from build123d import *

# Parameters (mm, degrees)
EXTRUDE_START            = -16
SKETCH_1_R               = 13
EXTRUDE_1_DEPTH          = 22
CUT_EXTRUDE_1_REACH      = 26.372
SKETCH_2_R               = 8
CUT_EXTRUDE_2_REACH      = 26.372
SKETCH_3_R               = 10
CUT_EXTRUDE_3_DEPTH      = 25.372115214
CUT_EXTRUDE_3_DEPTH_BACK = 25.372115214
SKETCH_4_R               = 3
SKETCH_4_R_2             = 2


with BuildPart() as part:
    # 草图1 → 凸台-拉伸1 (new body)
    with BuildSketch(Plane(origin=(0, 0, 0), x_dir=(1, 0, 0), z_dir=(0, 1, 0)).offset(EXTRUDE_START)):
        with Locations(Location((0, 0, 0), (0, 0, 270))):
            Circle(SKETCH_1_R)
    extrude(amount=EXTRUDE_1_DEPTH)

    # 草图2 → 切除-拉伸1 (cut, up to next)
    with BuildSketch(Plane(origin=(0, 0, 0), x_dir=(1, 0, 0), z_dir=(0, 1, 0)), mode=Mode.PRIVATE) as cut_extrude_1_sk1:
        with Locations(Location((0, 0, 0), (0, 0, 270))):
            Circle(SKETCH_2_R)
    cut_extrude_1_tool1 = extrude(cut_extrude_1_sk1.sketch, amount=CUT_EXTRUDE_1_REACH, mode=Mode.PRIVATE) & part.part
    add(cut_extrude_1_tool1.solids().sort_by_distance((0, 0, 0))[0], mode=Mode.SUBTRACT)

    # 草图3 → 切除-拉伸2 (cut, up to next)
    with BuildSketch(Plane(origin=(0, 0, 0), x_dir=(1, 0, 0), z_dir=(0, 1, 0)), mode=Mode.PRIVATE) as cut_extrude_2_sk1:
        with Locations(Location((0, 0, 0), (0, 0, 270))):
            Circle(SKETCH_3_R)
    cut_extrude_2_tool1 = extrude(cut_extrude_2_sk1.sketch, amount=-CUT_EXTRUDE_2_REACH, mode=Mode.PRIVATE) & part.part
    add(cut_extrude_2_tool1.solids().sort_by_distance((0, 0, 0))[0], mode=Mode.SUBTRACT)

    # 草图4 → 切除-拉伸3 (cut, two sides: drawn at the far end of the back side and taken through both)
    with BuildSketch(Plane.XY.offset(-CUT_EXTRUDE_3_DEPTH_BACK)):
        with Locations((0, -9)):
            Circle(SKETCH_4_R)
        with Locations((0, 3)):
            Circle(SKETCH_4_R_2)
    extrude(amount=CUT_EXTRUDE_3_DEPTH + CUT_EXTRUDE_3_DEPTH_BACK, mode=Mode.SUBTRACT)


solid = part.part
The listing builds one solid part. Answer for the finished solid, in the listing's coordinates (mm). A direction names the side the tool comes from. Round coordinates to 2 decimals unless told otherwise and drop trailing zeros. Order: outer loops, then holes, each group sorted by start corner. A loop starts at its lowest first (then second) coordinate and runs counter-clockwise, first axis right, second up. Notation, with made-up numbers: M 13,3.5 L 62,3.5 A16 cw 62,22.5 Z; hole C 1.25,76 d5. An arc over 180 degrees is marked long. Answer in a Markdown table with one row per item. Add a question column.
1) Determine the mould class of faces 3 (the face through (3, -7.89, 9.54)), 4 (the face through (-5, -5, 12)), 5 (the face through (0, 1, -10)) for opening direction Z: pulls with the +Z half, pulls with the -Z half, needs draft (parallel to the pull), parting line crosses it, or undercut.
2) Consider line 1 along Y through (x, z) = (0, 10.35); line 2 along X through (y, z) = (-9, -10.25); line 3 along X through (y, z) = (-4.25, 0). Determine where each line is inside the solid, lowest interval first. Write a range as from..to.
3) Flat-ended cylindrical pins translate along their axes: pin 1 Ø4 at (y, z) = (2.5, -10) entering from +X; pin 2 Ø4 at (x, y) = (5, -11.5) entering from +Z; pin 3 Ø1 at (x, y) = (8, -9) entering from -Z. Find the tip coordinate at first contact, or state that the pin passes through.
4) The part is cut by section B-B on y = -9. Determine the outline of the cut face in (x, z), plus the area to 3 significant figures.
5) Which of the six approach directions +Z, -Z, +X, -X, +Y, -Y give full straight-line access (tool end or side, diameter ignored) to faces 1 (the face through (8.2, 0, 0)), 2 (the face through (-3.06, 2.96, 7.39))?
6) The part is cut by section D-D on x = 4.75. Determine the outline of the cut face in (y, z).
7) The part is cut by section C-C on x = -1. Determine the outline of the cut face in (y, z).
8) The part is cut by section A-A on z = 0. Determine the outline of the cut face in (x, y), plus the area to 3 significant figures.
Findings below:
| question | item | result |
|---|---|---|
| 1 | face 3 | undercut |
| 1 | face 4 | parting line crosses it |
| 1 | face 5 | needs draft |
| 2 | line 1 | y = -16..-12, -6..1, 5..6 |
| 2 | line 2 | x = -8..-3, 3..8 |
| 2 | line 3 | x = -13..-10, 10..13 |
| 3 | pin 1 | stops at x = 10.25 |
| 3 | pin 2 | stops at z = 12.65 |
| 3 | pin 3 | stops at z = -10.62 |
| 4 | outline | M -3,-12.65 L -3,-9.54 A10 cw -3,9.54 L -3,12.65 A13 ccw Z; M 3,-12.65 A13 ccw 3,12.65 L 3,9.54 A10 cw 3,-9.54 Z |
| 4 | area | 180 mm² |
| 5 | face 1 | -Y |
| 5 | face 2 | +Y, -Y |
| 6 | outline | M -16,-12.1 L 6,-12.1 L 6,-6.44 L 0,-6.44 L 0,-8.8 L -16,-8.8 Z; M -16,8.8 L 0,8.8 L 0,6.44 L 6,6.44 L 6,12.1 L -16,12.1 Z |
| 7 | outline | M -16,-12.96 L -11.83,-12.96 L -11.83,-9.95 L -16,-9.95 Z; M -16,9.95 L -11.83,9.95 L -11.83,12.96 L -16,12.96 Z; M -6.17,-12.96 L 1.27,-12.96 L 1.27,-7.94 L 0,-7.94 L 0,-9.95 L -6.17,-9.95 Z; M -6.17,9.95 L 0,9.95 L 0,7.94 L 1.27,7.94 L 1.27,12.96 L -6.17,12.96 Z; M 4.73,-12.96 L 6,-12.96 L 6,-7.94 L 4.73,-7.94 Z; M 4.73,7.94 L 6,7.94 L 6,12.96 L 4.73,12.96 Z |
| 8 | outline | M -13,-16 L -10,-16 L -10,0 L -8,0 L -8,6 L -13,6 Z; M 8,0 L 10,0 L 10,-16 L 13,-16 L 13,6 L 8,6 Z |
| 8 | area | 156 mm² |
